from build123d import *

# Parameters (mm, degrees)
BOSS_EXTRUDE1_DEPTH = 30
BOSS_EXTRUDE2_DEPTH = 25
BOSS_EXTRUDE8_REACH = 304.903
SKETCH5_W           = 30
SKETCH5_H           = 30
BOSS_EXTRUDE9_DEPTH = 20


with BuildPart() as part:
    # Sketch1 → Boss-Extrude1 (new body)
    with BuildSketch(Plane.XY):
        Polygon((-60, 0), (-40, 0), (-40, 230), (40, 230), (40, 0), (60, 0), (60, 250), (-60, 250), align=None)
    extrude(amount=BOSS_EXTRUDE1_DEPTH)

    # Sketch4 → Boss-Extrude2 (add)
    with BuildSketch(Plane(origin=(0, 100, 0), x_dir=(-1, 0, 0), z_dir=(0, -1, 0))):
        with BuildLine():
            Line((-60, -30), (-75, -30))
            Line((-75, -30), (-75, 0))
            Line((-75, 0), (-105, 30))
            ThreePointArc((-105, 30), (-90, 45), (-75, 30))
            Line((-75, 30), (-30, 0))
            Line((-30, 0), (-30, -30))
            Line((-30, -30), (-60, -30))
        make_face()
    boss_extrude2 = extrude(amount=-BOSS_EXTRUDE2_DEPTH)

    # Mirror1: Boss-Extrude2 across plane
    add(boss_extrude2.mirror(Plane(origin=(0, 0, 0), x_dir=(0, 0, 1), z_dir=(1, 0, 0))))

    # Boss-Extrude8: up to this face of the body (flat: up to its plane)
    boss_extrude8_end = Plane(part.part.faces().sort_by_distance((60, 50, 15))[0])
    # Sketch5 → Boss-Extrude8 (add, up to the picked face)
    with BuildSketch(Plane.ZY.offset(60), mode=Mode.PRIVATE) as boss_extrude8_sk1:
        with Locations((45, 60)):
            Rectangle(SKETCH5_W, SKETCH5_H)
    boss_extrude8_tool1 = split(extrude(boss_extrude8_sk1.sketch, amount=-BOSS_EXTRUDE8_REACH, mode=Mode.PRIVATE), bisect_by=boss_extrude8_end, keep=Keep.BOTH, mode=Mode.PRIVATE)
    add(boss_extrude8_tool1.solids().sort_by(Axis((-60, 60, 45), (1, 0, 0)))[0])

    # Sketch6 → Boss-Extrude9 (add, symmetric)
    with BuildSketch(Plane(origin=(0, 0, 0), x_dir=(0, 0, -1), z_dir=(1, 0, 0))):
        with BuildLine():
            Line((-30, 230), (5, 230))
            Line((5, 230), (5, 250))
            ThreePointArc((5, 250), (10.857864376, 264.142135624), (25, 270))
            Line((25, 270), (45, 270))
            Line((45, 270), (45, 290))
            Line((45, 290), (-30, 290))
            Line((-30, 290), (-30, 230))
        make_face()
    extrude(amount=BOSS_EXTRUDE9_DEPTH, both=True)


solid = part.part
Design review of the part built by this model. Coordinates are the model's own, in mm. A direction names the side the tool comes from. Give positions to 0.01 mm unless a question says otherwise; leave off trailing zeros. Order: outer loops, then holes, each group sorted by start corner. A loop starts at its lowest first (then second) coordinate and runs counter-clockwise, first axis right, second up.
1. To check wall thickness, follow L1, parallel to X at y = 66, z = 26; L2, parallel to Y at x = 32, z = 20.5; L3, parallel to X at y = 111.5, z = 20. State the ranges of each line that lie inside material, in increasing order.
Solution:
L1: x = -60 to -40, 40 to 60
L2: y = 100 to 125, 230 to 250
L3: x = -75 to -30, 30 to 75
2. Add section B-B, the plane y = 141. State the section outline as (x, z) points.
Solution:
outline: (-60, 0) - (-40, 0) - (-40, 30) - (-60, 30) - close; (40, 0) - (60, 0) - (60, 30) - (40, 30) - close
3. Add section D-D, the plane x = -56. State the section outline as (y, z) points, then the cut area to 3 significant figures.
Solution:
outline: (0, 0) - (100, 0) - (100, -17.33) - (125, -17.33) - (125, 0) - (250, 0) - (250, 30) - (75, 30) - (75, 60) - (45, 60) - (45, 30) - (0, 30) - close
area: 8,830 mm2
4. Tool access review of faces 4 (the flat face through (-60, 188, 15)), 5 (the flat face through (75, 112, 15)), 6 (the flat face through (50, 22, 30)): name each direction out of +Z, -Z, +X, -X, +Y, -Y from which nothing blocks a thin tool from reaching the whole face with its end or side.
Solution:
face 4: +Z, -Z, -X, +Y
face 5: +Z, +X, +Y, -Y
face 6: +Z, +X, -X, -Y
5. For pin 1 Ø9 at (y, z) = (218.5, 19) entering from -X; pin 2 Ø3 at (x, z) = (20.5, 25.5) entering from -Y; pin 3 Ø16 at (x, y) = (-54, 64.5) entering from -Z; pin 4 Ø10 at (y, z) = (211, -8) entering from -X, all flat-tipped, find the tip position at first contact; note any pin that passes through.
Solution:
pin 1: stops at x = -60
pin 2: stops at y = 230
pin 3: stops at z = 0
pin 4: passes through
6. Mouldability with a two-part tool opening along Y and no side actions: class faces 1 (the flat face through (-1, 45, 45)), 2 (the flat face through (-90, 112, -15)), 3 (the flat face through (67, 125, -8)) as +Y half, -Y half, draft (parallel to the pull), parting line (faces both ways), or undercut.
Solution:
face 1: -Y half
face 2: draft
face 3: undercut
7. Add section A-A, the plane x = 6.5. State the section outline as (y, z) points.
Solution:
outline: (45, 30) - (75, 30) - (75, 60) - (45, 60) - close; (230, -5) - (250, -5) arc R20 cw to (270, -25) - (270, -45) - (290, -45) - (290, 30) - (230, 30) - close
8. Add section C-C, the plane z = 4.5. State the section outline as (x, y) points.
Solution:
outline: (-75, 100) - (-60, 100) - (-60, 0) - (-40, 0) - (-40, 100) - (-30, 100) - (-30, 125) - (-40, 125) - (-40, 230) - (40, 230) - (40, 125) - (30, 125) - (30, 100) - (40, 100) - (40, 0) - (60, 0) - (60, 100) - (75, 100) - (75, 125) - (60, 125) - (60, 250) - (20, 250) - (20, 290) - (-20, 290) - (-20, 250) - (-60, 250) - (-60, 125) - (-75, 125) - close
